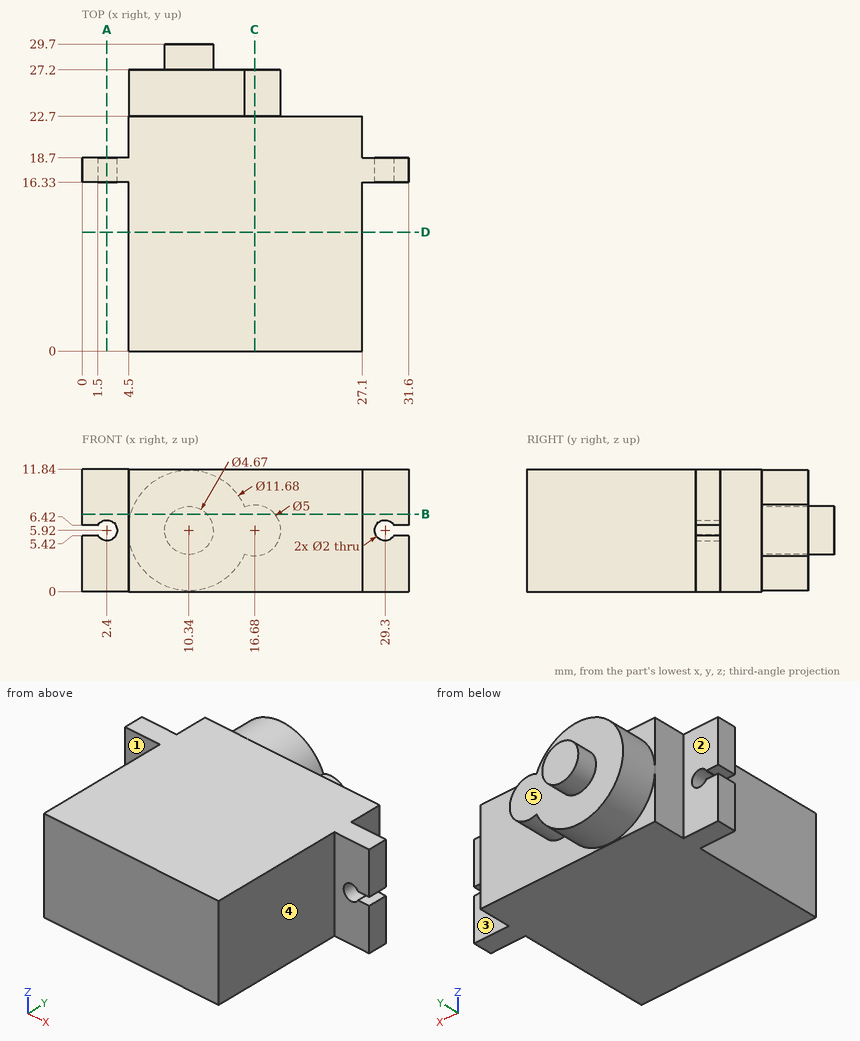
Part print with two shaded views. Sizes in mm from the minimum x, y, z corner. A direction names the side the tool comes from. Round coordinates to 2 decimals unless told otherwise and drop trailing zeros. Write each loop counter-clockwise with the first axis right and the second up, starting at its lowest first coordinate (ties: lowest second). Pieces come first, ordered by that corner, then holes. Notation, with made-up numbers: (65.5, 71) - (109.5, 71) arc R24 cw to (109.5, 105) - close; hole circle Ø9 at (71.5, 68.5). An arc over 180 degrees is marked (long way). Answer as CSV lines item,"result".
Q1. Drop flat-ended pins along their axis: pin 1 (2 mm diameter, centred on y = 21.5, z = 6.5, fed in from -X); pin 2 (4 mm diameter, centred on y = 10, z = 10.5, fed in from +X); pin 3 (1.8 mm diameter, centred on x = 2.4, z = 5.92, fed in from -Y); pin 4 (2.5 mm diameter, centred on x = 29.3, z = 5.92, fed in from +Y). Give the stop position or say it passes through.
Report:
pin 1,"stops at x = 4.5"
pin 2,"stops at x = 27.1"
pin 3,"passes through"
pin 4,"stops at y = 18.7"
Q2. Drill centre lines: probe 1 along Z at (x, y) = (29.3, 18.1); probe 2 along Y at (x, z) = (25, 2.25); probe 3 along X at (y, z) = (22.25, 11). Where is each one in solid material? Low to high. Write a range as [from, to].
Report:
probe 1,"z = [0, 4.92], [6.92, 11.84]"
probe 2,"y = [0, 22.7]"
probe 3,"x = [4.5, 27.1]"
Q3. Cut at C-C (x = 16.68). Write the cut outline in (y, z), and give its area (3 significant figures).
Report:
outline,"(0, 0) - (22.7, 0) - (22.7, 3.42) - (27.2, 3.42) - (27.2, 8.42) - (22.7, 8.42) - (22.7, 11.84) - (0, 11.84) - close"
area,"291 mm^2"
Q4. Cut at B-B (z = 7.5). Write the cut outline in (x, y), and give its area (3 significant figures).
Report:
outline,"(0, 16.33) - (4.5, 16.33) - (4.5, 0) - (27.1, 0) - (27.1, 16.33) - (31.6, 16.33) - (31.6, 18.7) - (27.1, 18.7) - (27.1, 22.7) - (18.62, 22.7) - (18.62, 27.2) - (12.06, 27.2) - (12.06, 29.7) - (8.62, 29.7) - (8.62, 27.2) - (4.72, 27.2) - (4.72, 22.7) - (4.5, 22.7) - (4.5, 18.7) - (0, 18.7) - close"
area,"605 mm^2"
Q5. Cut at A-A (x = 2.4). Write the cut outline in (y, z).
Report:
outline,"(16.33, 0) - (18.7, 0) - (18.7, 4.92) - (16.33, 4.92) - close; (16.33, 6.92) - (18.7, 6.92) - (18.7, 11.84) - (16.33, 11.84) - close"
Q6. Cut at D-D (y = 11.5). Write the cut outline in (x, z), and give its area (3 significant figures).
Report:
outline,"(4.5, 0) - (27.1, 0) - (27.1, 11.84) - (4.5, 11.84) - close"
area,"268 mm^2"
Q7. Tool access for the marked faces 1, 2, 3, 4 and 5: list every direction of +Z, -Z, +X, -X, +Y, -Y with a clear straight run to the whole face (end or side of a thin tool).
Report:
face 1,"+Z, -Z, -X, -Y"
face 2,"+Z, -Z, -X, +Y"
face 3,"+Z, -Z, +X, +Y"
face 4,"+Z, -Z, +X, -Y"
face 5,"+Y"
